```python
from build123d import *

# Parameters (mm, degrees)
F1_DEPTH = 6
F3_DEPTH = 4


with BuildPart() as f1:
    # F0 (on Top) → F1 (new body)
    with BuildSketch(Plane.XY):
        with BuildLine():
            ThreePointArc((45.172989, -80), (48.001416, -78.828427), (49.172989, -76))
            Line((49.172989, -76), (49.172989, -30))
            Line((49.172989, -30), (24, 0))
            Line((24, 0), (0, 0))
            Line((0, 0), (25.172989, -30))
            Line((25.172989, -30), (25.172989, -76))
            ThreePointArc((25.172989, -76), (26.344562, -78.828427), (29.172989, -80))
            Line((29.172989, -80), (45.172989, -80))
        make_face()
    extrude(amount=F1_DEPTH)

    # F2 (on face) → F3 (cut)
    with BuildSketch(Plane.XY.offset(6)):
        Polygon((4, 0), (29.172989, -30), (45.172989, -30), (20, 0), align=None)
    extrude(amount=-F3_DEPTH, mode=Mode.SUBTRACT)


solid = f1.part
```
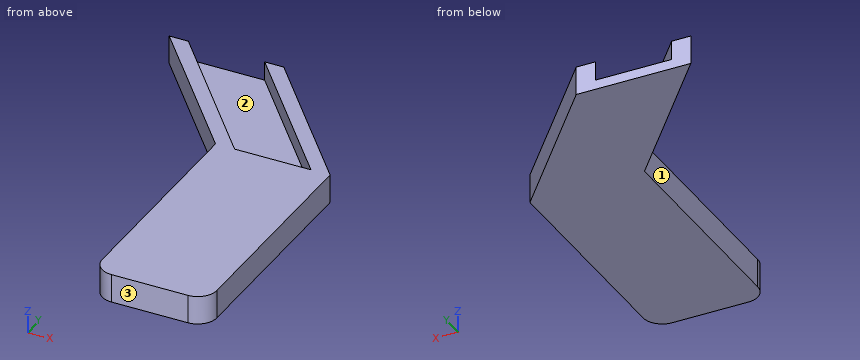
Model file for the job. Use its own axes, mm. Face numbers are marked on the shaded views. A direction names the side the tool comes from. Give positions to 0.01 mm unless a question says otherwise; leave off trailing zeros. Loops run counter-clockwise (first coordinate to the right, second up) from the corner with the lowest first, then second, coordinate; pieces in that order, holes last. Notation, with made-up numbers: (20, -32) -> (68, -32) arc R15 cw to (68, -14) -> close; hole circle Ø7 at (41.5, -0.75). An arc over 180 degrees is marked (long way). Write each question's results on one line, items separated by ' | '.
(1) Cut at C-C on x = 6. List the corners of the cut face in (y, z).
Geometry results:
outline: (-7.15, 0) -> (0, 0) -> (0, 2) -> (-2.38, 2) -> (-2.38, 6) -> (-7.15, 6) -> close
(2) Tool access for the marked faces 1, 2 and 3: list every direction of +Z, -Z, +X, -X, +Y, -Y with a clear straight run to the whole face (end or side of a thin tool).
Geometry results:
face 1: +Z, -Z, -X, -Y | face 2: +Z | face 3: +Z, -Z, +X, -X, -Y
(3) Flat gauge pins, fed straight in: pin 1 Ø1.8 at (y, z) = (-56.5, 3.5) entering from -X; pin 2 Ø2 at (x, z) = (36.5, 4) entering from +Y. Where does each tip first touch, or does it go through?
Geometry results:
pin 1: stops at x = 25.17 | pin 2: stops at y = -13.71
(4) Cut at A-A on z = 0.95. List the corners of the cut face in (x, y).
Geometry results:
outline: (0, 0) -> (25.17, -30) -> (25.17, -76) arc R4 ccw to (29.17, -80) -> (45.17, -80) arc R4 ccw to (49.17, -76) -> (49.17, -30) -> (24, 0) -> close
(5) Probe line 1 along X through (y, z) = (-45, 5.1); line 2 along Y through (x, z) = (32.5, 2.4); line 3 along Y through (x, z) = (36, 2.55). List the from-to ranges inside material, lowest first.
Geometry results:
line 1: x = 25.17 to 49.17 | line 2: y = -80 to -30, -14.9 to -10.13 | line 3: y = -80 to -30, -19.07 to -14.3
(6) Cut at B-B on y = -7.5. List the corners of the cut face in (x, z), and give its area (3 significant figures).
Geometry results:
outline: (6.29, 0) -> (30.29, 0) -> (30.29, 6) -> (26.29, 6) -> (26.29, 2) -> (10.29, 2) -> (10.29, 6) -> (6.29, 6) -> close | area: 80.0 mm²
(7) Cut at D-D on y = -37. List the corners of the cut face in (x, z), and give its area (3 significant figures).
Geometry results:
outline: (25.17, 0) -> (49.17, 0) -> (49.17, 6) -> (25.17, 6) -> close | area: 144 mm²
